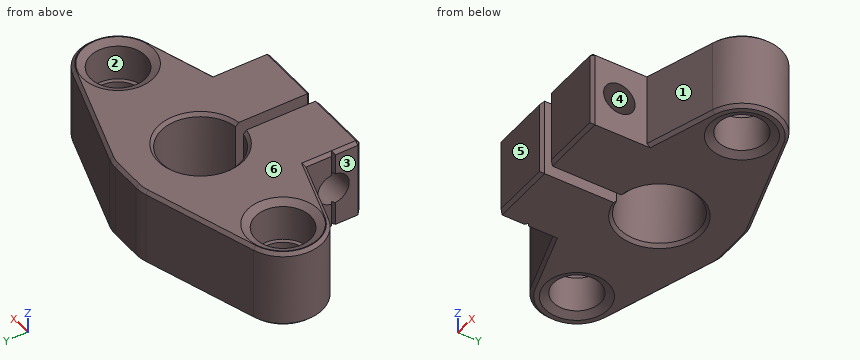
```python
from build123d import *

# Parameters (mm, degrees)
BOSS_EXTRUDE1_DEPTH             = 10
CUT_EXTRUDE1_DEPTH              = 28.408940147
CUT_EXTRUDE2_DEPTH              = 28.408940147
DRAFT1_ANGLE                    = 30
SKETCH4_W                       = 5
SKETCH4_H                       = 10
SKETCH5_W                       = 2
SKETCH5_H                       = 20.25
F_4_0_4_DIAMETER_HOLE2_D        = 4
F_4_0_4_DIAMETER_HOLE2_DEPTH    = 20.25
M7X1_0_TAPPED_HOLE1_D           = 6
M7X1_0_TAPPED_HOLE1_CBORE_D     = 7
M7X1_0_TAPPED_HOLE1_CBORE_DEPTH = 5
FILLET1_R                       = 5
CHAMFER1_SIZE                   = 1
CHAMFER1_SIZE2                  = 0.487732589
CHAMFER2_SIZE                   = 0.4
CHAMFER3_SIZE                   = 1
CHAMFER3_SIZE2                  = 0.487732589


with BuildPart() as part:
    # Sketch1 → Boss-Extrude1 (new body)
    with BuildSketch(Plane.XY.offset(10)):
        with BuildLine():
            Line((-9, -7.5), (-9, -14.5))
            Line((-9, -14.5), (9, -14.5))
            Line((9, -14.5), (9, -7.5))
            Line((9, -7.5), (17.529062862, -4.760458672))
            ThreePointArc((17.529062862, -4.760458672), (21, 0), (17.529062862, 4.760458672))
            Line((17.529062862, 4.760458672), (2.773364341, 9.5))
            Line((2.773364341, 9.5), (-2.773364341, 9.5))
            Line((-2.773364341, 9.5), (-17.529062862, 4.760458672))
            ThreePointArc((-17.529062862, 4.760458672), (-21, 0), (-17.529062862, -4.760458672))
            Line((-17.529062862, -4.760458672), (-9, -7.5))
        make_face()
    extrude(amount=-BOSS_EXTRUDE1_DEPTH)

    # Sketch2 → Cut-Extrude1 (cut, through all)
    with BuildSketch(Plane(origin=(0, 0, 0), x_dir=(-1, 0, 0), z_dir=(0, 0, -1))):
        Polygon((9, -11.230940108), (9, -10.769059892), (8.2, -10.769059892), align=None)
    extrude(amount=-CUT_EXTRUDE1_DEPTH, mode=Mode.SUBTRACT)

    # Sketch3 → Cut-Extrude2 (cut, through all)
    with BuildSketch(Plane(origin=(0, 0, 0), x_dir=(-1, 0, 0), z_dir=(0, 0, -1))):
        with BuildLine():
            Line((0.75, -14.5), (0.75, -4.943429983))
            ThreePointArc((0.75, -4.943429983), (0, -5), (-0.75, -4.943429983))
            Line((-0.75, -4.943429983), (-0.75, -14.5))
            Line((-0.75, -14.5), (0.75, -14.5))
        make_face()
    extrude(amount=-CUT_EXTRUDE2_DEPTH, mode=Mode.SUBTRACT)

    # Draft1
    draft1_faces = [part.faces().sort_by_distance(p)[0] for p in [
        (-8.6, -10.769059892, 5),
    ]]
    draft(draft1_faces, Plane(origin=(-9, -7.5, 0), x_dir=(0, 0, -1), z_dir=(-1, 0, 0)), DRAFT1_ANGLE)

    # Sketch4 → Cut-Revolve1 (revolve, cut)
    with BuildSketch(Plane.XZ):
        with Locations((2.5, 5)):
            Rectangle(SKETCH4_W, SKETCH4_H)
    revolve(axis=Axis((0, 0, 10), (0, 0, -1)), mode=Mode.SUBTRACT)

    # Sketch5 → Ø4.0 (4) Diameter Hole1 (revolve, cut)
    with BuildSketch(Plane(origin=(-0.75, -11, 5), x_dir=(0, 0, -1), z_dir=(0, 1, 0))):
        with Locations((1, 10.125)):
            Rectangle(SKETCH5_W, SKETCH5_H)
    revolve(axis=Axis((5.6, -11, 5), (-1, 0, 0)), mode=Mode.SUBTRACT)

    # Ø4.0 (4) Diameter Hole2
    with Locations(Plane.ZY.offset(-0.75)):
        with Locations((5, -11)):
            Hole(F_4_0_4_DIAMETER_HOLE2_D / 2, depth=F_4_0_4_DIAMETER_HOLE2_DEPTH)

    # M7x1.0 Tapped Hole1 (through all)
    with Locations(Plane.XY.offset(10)):
        with Locations((-16, 0), (16, 0)):
            CounterBoreHole(M7X1_0_TAPPED_HOLE1_D / 2, M7X1_0_TAPPED_HOLE1_CBORE_D / 2, M7X1_0_TAPPED_HOLE1_CBORE_DEPTH)

    # Fillet1
    fillet1_edges = [part.edges().sort_by_distance(p)[0] for p in [
        (-2.773364341, 9.5, 5),
        (2.773364341, 9.5, 5),
    ]]
    fillet(fillet1_edges, radius=FILLET1_R)

    # Chamfer1
    chamfer1_edges = [part.edges().sort_by_distance(p)[0] for p in [
        (12.5, 0, 10),
        (-19.5, 0, 10),
    ]]
    chamfer1_side = [part.faces().sort_by_distance(p)[0] for p in [
        (0, 9.016264535, 10),
    ]]
    chamfer(chamfer1_edges, length=CHAMFER1_SIZE, length2=CHAMFER1_SIZE2, reference=chamfer1_side[0])

    # Chamfer2
    chamfer2_edges = [part.edges().sort_by_distance(p)[0] for p in [
        (13.264531431, -6.130229336, 0),
        (21, 0, 0),
        (10.524097746, 7.010458672, 0),
        (2.763925905, 9.439751682, 0),
        (0, 9.5, 0),
        (-2.763925905, 9.439751682, 0),
        (-10.524097746, 7.010458672, 0),
        (-13.264531431, -6.130229336, 0),
        (-21, 0, 0),
        (-9, -9.134529946, 10),
        (-13.264531431, -6.130229336, 10),
        (-21, 0, 10),
        (-10.524097746, 7.010458672, 10),
        (-2.763925905, 9.439751682, 10),
        (0, 9.5, 10),
        (2.763925905, 9.439751682, 10),
        (10.524097746, 7.010458672, 10),
        (21, 0, 10),
        (13.264531431, -6.130229336, 10),
        (9, -11, 10),
        (4.875, -14.5, 10),
        (9, -14.5, 5),
        (0.75, -14.5, 5),
        (4.875, -14.5, 0),
        (0, 5, 10),
        (-9, -12.865470054, 10),
        (-9, -14.5, 5),
        (-4.875, -14.5, 0),
        (-0.75, -14.5, 5),
        (-4.875, -14.5, 10),
        (0, 5, 0),
    ]]
    chamfer(chamfer2_edges, length=CHAMFER2_SIZE - 0.0001)  # a hair under: the kernel refuses the full size

    # Chamfer3
    chamfer3_edges = [part.edges().sort_by_distance(p)[0] for p in [
        (19, 0, 0),
        (-13, 0, 0),
    ]]
    chamfer3_side = [part.faces().sort_by_distance(p)[0] for p in [
        (4.875, -13.627267497, 0),
    ]]
    chamfer(chamfer3_edges, length=CHAMFER3_SIZE, length2=CHAMFER3_SIZE2, reference=chamfer3_side[0])


solid = part.part
```
Part model, mm, in its own coordinate system. Face numbers are marked on the shaded views. A direction names the side the tool comes from. Give positions to 0.01 mm unless a question says otherwise; leave off trailing zeros. Order: outer loops, then holes, each group sorted by start corner. A loop starts at its lowest first (then second) coordinate and runs counter-clockwise, first axis right, second up. Notation, with made-up numbers: M 61,13.25 L 81,13.25 A28 cw 81,43.25 Z; hole C 63,-9 d2. An arc over 180 degrees is marked long. Use a Markdown table: item, result. Add a question column.
(1) Saw through at B-B, the plane y = -8.5. Give the cut face in (x, z).
(2) Saw through at A-A, the plane z = 1.5. Give the cut face in (x, y).
(3) Saw through at C-C, the plane z = 6.25. Give the number of separate pieces and of enclosed holes in the cut face, and give its area (3 significant figures).
(4) Drop flat-ended pins along their axis: P1, Ø1.8, axis at y = -8.5, z = 5, coming from the -X side; P2, Ø2, axis at x = -10.5, y = -10, coming from the -Z side; P3, Ø5.5, axis at x = 16, y = 0.5, coming from the +Z side; P4, Ø4.5, axis at y = -11, z = 5, coming from the +X side. Give the stop position or say it passes through.
(5) Probe line 1 along Z through (x, y) = (-5.25, -11); line 2 along X through (y, z) = (-10.75, 1.25); line 3 along X through (y, z) = (0.5, 2.75). List the from-to ranges inside material, lowest first. Write a range as [from, to].
(6) Saw through at D-D, the plane x = -6. Give the cut face in (y, z), and give its area (3 significant figures).
(7) Mould opens along Z. For the marked faces 4, 5 and 6 say: +Z half, -Z half, draft (parallel to the pull), parting line (faces both ways), or undercut.
(8) 3-axis set-ups, long thin cutter, end or side, ignore diameter. For the marked faces 1, 2 and 3: which of +Z, -Z, +X, -X, +Y, -Y reach the whole face in a straight line?
Answer key:
| question | item | result |
|---|---|---|
| 1 | outline | M -9,0 L -0.75,0 L -0.75,10 L -8.6,10 L -9,9.6 Z; M 0.75,0 L 9,0 L 9,9.6 L 8.6,10 L 0.75,10 Z |
| 2 | outline | M -17.53,-4.76 L -9,-7.5 L -9,-10.77 L -8.6,-11 L -9,-11.23 L -9,-14.1 L -8.6,-14.5 L -1.15,-14.5 L -0.75,-14.1 L -0.75,-4.94 A5 cw long 0.75,-4.94 L 0.75,-14.1 L 1.15,-14.5 L 8.6,-14.5 L 9,-14.1 L 9,-7.5 L 17.53,-4.76 A5 ccw 17.53,4.76 L 3.52,9.26 A5 ccw 1.99,9.5 L -1.99,9.5 A5 ccw -3.52,9.26 L -17.53,4.76 A5 ccw Z; hole C -16,0 d6; hole C 16,0 d6 |
| 3 | separate pieces | 3 |
| 3 | enclosed holes | 2 |
| 3 | area | 455 mm^2 |
| 4 | P1 | x = -9 |
| 4 | P2 | through |
| 4 | P3 | z = 5 |
| 4 | P4 | x = 9 |
| 5 | line 1 | [0, 3], [7, 10] |
| 5 | line 2 | [-9, -0.75], [0.75, 9] |
| 5 | line 3 | [-20.97, -18.96], [-13.04, -4.97], [4.97, 13.04], [18.96, 20.97] |
| 6 | outline | M -14.5,0.4 L -14.1,0 L 8.04,0 L 8.46,0.4 L 8.46,9.6 L 8.04,10 L -14.1,10 L -14.5,9.6 Z; hole C -11,5 d4 |
| 6 | area | 217 mm^2 |
| 7 | face 4 | undercut |
| 7 | face 5 | draft |
| 7 | face 6 | +Z half |
| 8 | face 1 | +Z, -Z, +X, -Y |
| 8 | face 2 | +Z |
| 8 | face 3 | +Z, -Z, -X, -Y |
